Check sheet for the drawn part. Datum: minimum x, y, z corner. Units: mm. A direction names the side the tool comes from. Give positions to 0.01 mm unless a question says otherwise; leave off trailing zeros. Order: outer loops, then holes, each group sorted by start corner. A loop starts at its lowest first (then second) coordinate and runs counter-clockwise, first axis right, second up. Notation, with made-up numbers: (55.5, 8) -> (105.5, 8) arc R28 cw to (105.5, 29) -> close; hole circle Ø11 at (-25, 20). An arc over 180 degrees is marked (long way). One line per question, with ' | ' between items. Start each with the question number.
Q1. Section check D-D on x = 12. Record the cut outline in (y, z).
Q2. Go/stop test with flat-tipped pins: pin 1 (6.5 mm diameter, centred on x = 7.5, z = 6.5, fed in from -Y); pin 2 (5 mm diameter, centred on x = 3, y = 23, fed in from -Z); pin 3 (6 mm diameter, centred on x = 11.5, z = 10, fed in from -Y); pin 4 (1 mm diameter, centred on x = 10.5, z = 2.5, fed in from -Y). Record where each tip stops, or that it passes through.
Q3. Section check C-C on y = 22. Record the cut outline in (x, z).
Q4. Material ranges on probe 1 along Y at (x, z) = (11.25, 3); probe 2 along Y at (x, z) = (8, 9.25); probe 3 along Z at (x, y) = (7.25, 44), recorded low to high. Write a range as [from, to].
Q5. Access from +Z, -Z, +X, -X, +Y, -Y to the whole of each face (thin tool, end or side, straight path). Record for the marked faces 1, 2 and 3.
Q6. Section check A-A on x = 6.5. Record the cut outline in (y, z).
Q7. Section check B-B on z = 4.5. Record the cut outline in (x, y) (1 decimal).
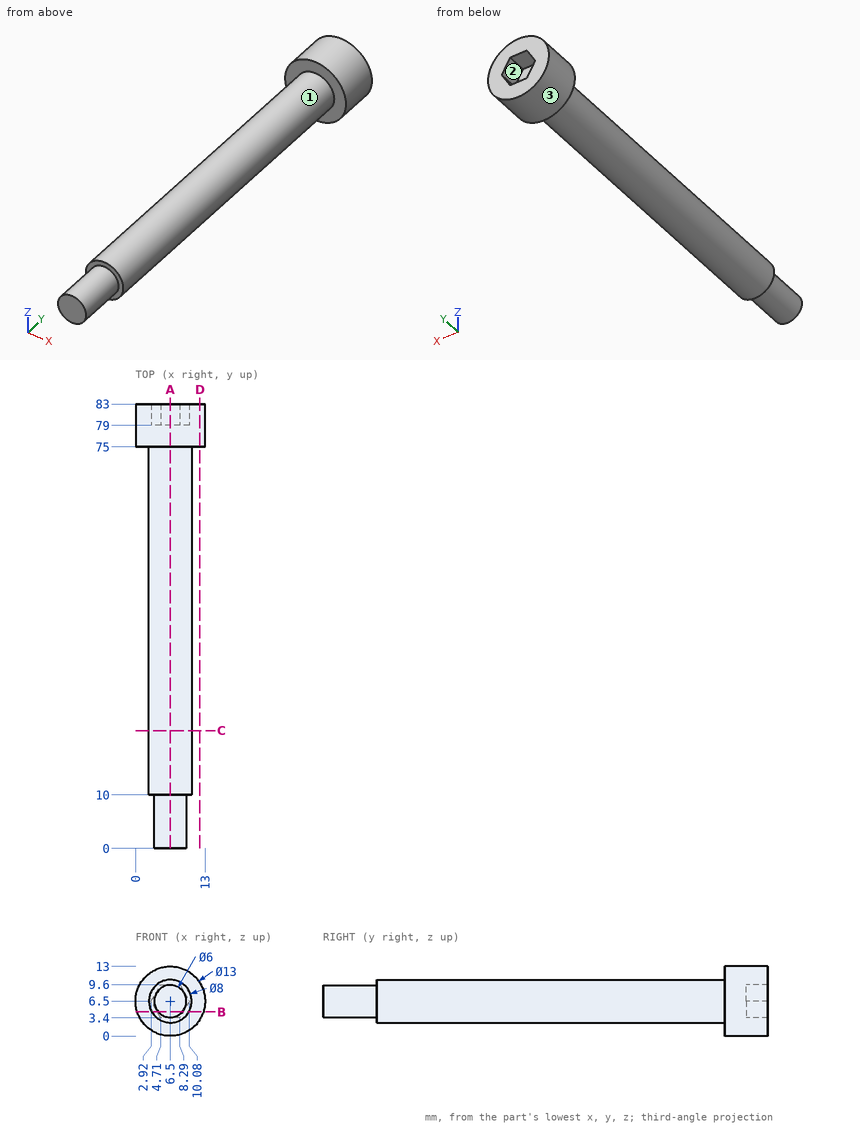
Filled in:
1) outline: (75, 3.04) -> (83, 3.04) -> (83, 9.96) -> (75, 9.96) -> close
2) pin 1: y = 0 | pin 2: z = 2.63 | pin 3: y = 10 | pin 4: y = 75
3) outline: circle Ø8 at (6.5, 6.5)
4) probe 1: [75, 83] | probe 2: [10, 79] | probe 3: [2.57, 10.43]
5) face 1: -Y | face 2: +Y | face 3: +Y, -Y
6) outline: (0, 3.5) -> (10, 3.5) -> (10, 2.5) -> (75, 2.5) -> (75, 0) -> (83, 0) -> (83, 3.4) -> (79, 3.4) -> (79, 9.6) -> (83, 9.6) -> (83, 13) -> (75, 13) -> (75, 10.5) -> (10, 10.5) -> (10, 9.5) -> (0, 9.5) -> close
7) outline: (0.3, 75) -> (3, 75) -> (3, 10) -> (4.3, 10) -> (4.3, 0) -> (8.7, 0) -> (8.7, 10) -> (10, 10) -> (10, 75) -> (12.7, 75) -> (12.7, 83) -> (8.9, 83) -> (8.9, 79) -> (4.1, 79) -> (4.1, 83) -> (0.3, 83) -> close
